from build123d import *

# Parameters (mm, degrees)
EXTRUDE_446_DEPTH      = 4.5
EXTRUDE_871_DEPTH      = 2.4
SKETCH_7_R             = 1.25
SKETCH_7_R_2           = 2.5
CUT_EXTRUDE_1133_DEPTH = 3
CHAMFER_1178_SIZE      = 1.5
EXTRUDE_START          = 4.5
SKETCH_8_R             = 2.85
SKETCH_8_R_2           = 1.25
EXTRUDE_1547_DEPTH     = 4.5
SKETCH_9_R             = 1.65
CUT_EXTRUDE_1826_DEPTH = 3
SKETCH_13_R            = 1.2
CUT_EXTRUDE_2013_DEPTH = 5
CUT_EXTRUDE_START      = -7
SKETCH_14_R            = 1.2
CUT_EXTRUDE_2216_DEPTH = 7
FILLET_2261_R          = 2


with BuildPart() as part:
    # Эскиз1 → Extrude 446 (new body)
    with BuildSketch(Plane.XY):
        with BuildLine():
            ThreePointArc((-48.184740917, 154.510381185), (-49.352687792, 153.677592944), (-49.8, 152.314674038))
            Line((-49.8, 152.314674038), (-49.8, 88.338690467))
            ThreePointArc((-49.8, 88.338690467), (-48.67998968, 86.364450269), (-46.41076143, 86.312966069))
            ThreePointArc((-46.41076143, 86.312966069), (-8.509697807, 97.629257558), (30.777662843, 93.040971394))
            ThreePointArc((30.777662843, 93.040971394), (32.846964094, 93.360279245), (33.8, 95.224598888))
            Line((33.8, 95.224598888), (33.8, 156.408950918))
            ThreePointArc((33.8, 156.408950918), (33.279664307, 157.865932371), (31.954091345, 158.663679516))
            ThreePointArc((31.954091345, 158.663679516), (-8.376811335, 161.632472551), (-48.184740917, 154.510381185))
        make_face()
        with BuildLine():
            Line((-47.4, 152.241091851), (-47.4, 88.505842281))
            ThreePointArc((-47.4, 88.505842281), (-8.703725392, 100.021444112), (31.4, 95.362907453))
            Line((31.4, 95.362907453), (31.4, 156.32706115))
            ThreePointArc((31.4, 156.32706115), (-8.256741868, 159.235474256), (-47.4, 152.241091851))
        make_face(mode=Mode.SUBTRACT)
    extrude(amount=-EXTRUDE_446_DEPTH)

    # Эскиз2 → Extrude 871 (add)
    with BuildSketch(Plane.XY):
        with BuildLine():
            Line((-52.4, 152.314674038), (-52.4, 88.338690467))
            ThreePointArc((-52.4, 88.338690467), (-50.013891057, 84.132700481), (-45.179448263, 84.023016749))
            ThreePointArc((-45.179448263, 84.023016749), (-8.283928985, 95.039078329), (29.961107796, 90.572522923))
            ThreePointArc((29.961107796, 90.572522923), (34.369619156, 91.252787475), (36.4, 95.224598888))
            Line((36.4, 95.224598888), (36.4, 156.408950918))
            ThreePointArc((36.4, 156.408950918), (35.291458741, 159.512954882), (32.467411995, 161.212503148))
            ThreePointArc((32.467411995, 161.212503148), (-8.511379087, 164.228987816), (-48.958795866, 156.992484917))
            ThreePointArc((-48.958795866, 156.992484917), (-51.447030513, 155.218283882), (-52.4, 152.314674038))
        make_face()
    extrude(amount=EXTRUDE_871_DEPTH)

    # Эскиз7 → Cut-Extrude 1133 (cut)
    with BuildSketch(Plane(origin=(0, 0, 0), x_dir=(-1, 0, 0), z_dir=(0, 0, -1))):
        with Locations((-29.451383649, 150.200294851)):
            Circle(SKETCH_7_R)
        with Locations((45.554851126, 150.200369953)):
            Circle(SKETCH_7_R)
        with Locations((45.55089452, 119.209232592)):
            Circle(SKETCH_7_R)
        with Locations((-29.454420734, 119.20872198)):
            Circle(SKETCH_7_R)
        with Locations((0, 155)):
            Circle(SKETCH_7_R_2)
    extrude(amount=-CUT_EXTRUDE_1133_DEPTH, mode=Mode.SUBTRACT)

    # Chamfer 1178
    chamfer_1178_edges = [part.edges().sort_by_distance(p)[0] for p in [
        (30.704420734, 119.20872198, 2.4),
        (-44.30089452, 119.209232592, 2.4),
        (-44.304851126, 150.200369953, 2.4),
        (30.701383649, 150.200294851, 2.4),
    ]]
    chamfer(chamfer_1178_edges, length=CHAMFER_1178_SIZE)

    # Эскиз8 → Extrude 1547 (add)
    # profile 1 of 4: a face of its own
    with BuildSketch(Plane(origin=(0, 0, 0), x_dir=(-1, 0, 0), z_dir=(0, 0, -1)).offset(EXTRUDE_START)):
        with Locations((-29.454420734, 119.20872198)):
            Circle(SKETCH_8_R)
        with Locations((-29.454420734, 119.20872198)):
            Circle(SKETCH_8_R_2, mode=Mode.SUBTRACT)
    # profile 2 of 4: a face of its own
    with BuildSketch(Plane(origin=(0, 0, 0), x_dir=(-1, 0, 0), z_dir=(0, 0, -1)).offset(EXTRUDE_START)):
        with Locations((-29.451383649, 150.200294851)):
            Circle(SKETCH_8_R)
        with Locations((-29.451383649, 150.200294851)):
            Circle(SKETCH_8_R_2, mode=Mode.SUBTRACT)
    # profile 3 of 4: a face of its own
    with BuildSketch(Plane(origin=(0, 0, 0), x_dir=(-1, 0, 0), z_dir=(0, 0, -1)).offset(EXTRUDE_START)):
        with Locations((45.55089452, 119.209232592)):
            Circle(SKETCH_8_R)
        with Locations((45.55089452, 119.209232592)):
            Circle(SKETCH_8_R_2, mode=Mode.SUBTRACT)
    # profile 4 of 4: a face of its own
    with BuildSketch(Plane(origin=(0, 0, 0), x_dir=(-1, 0, 0), z_dir=(0, 0, -1)).offset(EXTRUDE_START)):
        with Locations((45.554851126, 150.200369953)):
            Circle(SKETCH_8_R)
        with Locations((45.554851126, 150.200369953)):
            Circle(SKETCH_8_R_2, mode=Mode.SUBTRACT)
    extrude(amount=-EXTRUDE_1547_DEPTH)

    # Эскиз9 → Cut-Extrude 1826 (cut)
    with BuildSketch(Plane(origin=(0, 0, 0), x_dir=(-1, 0, 0), z_dir=(0, 0, -1))):
        with Locations((-28.380750513, 99.381741539)):
            Circle(SKETCH_9_R)
        with Locations((44.512478568, 93.278276156)):
            Circle(SKETCH_9_R)
        with Locations((-19.894937989, 155.969982116)):
            Circle(SKETCH_9_R)
        with Locations((18.78344627, 156.107738518)):
            Circle(SKETCH_9_R)
    extrude(amount=-CUT_EXTRUDE_1826_DEPTH, mode=Mode.SUBTRACT)

    # Эскиз13 → Cut-Extrude 2013 (cut)
    with BuildSketch(Plane.ZY.offset(49.8)):
        with Locations((-2.25, 144.314674038)):
            Circle(SKETCH_13_R)
        with Locations((-2.25, 91.438690467)):
            Circle(SKETCH_13_R)
    extrude(amount=-CUT_EXTRUDE_2013_DEPTH, mode=Mode.SUBTRACT)

    # Эскиз14 → Cut-Extrude 2216 (cut)
    with BuildSketch(Plane(origin=(33.8, 0, 0), x_dir=(0, 0, -1), z_dir=(1, 0, 0)).offset(CUT_EXTRUDE_START)):
        with Locations(Location((2.25, 144.314674038, 0), (0, 0, 180))):
            Circle(SKETCH_14_R)
        with Locations(Location((2.25, 103.724598888, 0), (0, 0, 90))):
            Circle(SKETCH_14_R)
    extrude(amount=CUT_EXTRUDE_2216_DEPTH, mode=Mode.SUBTRACT)

    # Fillet 2261
    # the kernel refuses this fillet: 2 mm, written as the material it adds along each edge
    with BuildSketch(Plane(origin=(-44.944004027, 152.98413823, -4.5), x_dir=(0.9624896485032316, 0.2713184043225332, 0), z_dir=(0, 0, 1))) as fillet_2261_piece_1:
        with BuildLine():
            CenterArc((3.479493085, -1.99987944), FILLET_2261_R, 89.370889764, 96.709553608)
            ThreePointArc((1.490744771, -2.21172878), (1.020072901, -0.920711328), (0, 0))
            ThreePointArc((0, 0), (1.750726367, 0.009611624), (3.501452734, 0))
        make_face()
    extrude(amount=4.5)
    with BuildSketch(Plane(origin=(31.4, 156.32706115, 0), x_dir=(0, -1, 0), z_dir=(0, 0, -1))) as fillet_2261_piece_2:
        with BuildLine():
            CenterArc((1.646899326, 2), FILLET_2261_R, 190.761817139, 79.238182861)
            ThreePointArc((-0.317924487, 1.626546679), (-0.16107556, 0.812860271), (0, 0))
            Line((0, 0), (1.646899326, 0))
        make_face()
    extrude(amount=4.5)
    with BuildSketch(Plane(origin=(31.4, 95.362907453, 0), x_dir=(0, 1, 0), z_dir=(0, 0, -1))) as fillet_2261_piece_3:
        with BuildLine():
            CenterArc((2.725225415, -2), FILLET_2261_R, 90, 106.685074195)
            ThreePointArc((0.809430773, -2.574221986), (0.413364342, -1.284391441), (0, 0))
            Line((0, 0), (2.725225415, 0))
        make_face()
    extrude(amount=4.5)
    with BuildSketch(Plane(origin=(-47.4, 88.505842281, 0), x_dir=(0.889056274455369, 0.45779792578335204, 0), z_dir=(0, 0, -1))) as fillet_2261_piece_4_section:
        with BuildLine():
            CenterArc((3.279293139, -1.999738508), FILLET_2261_R, 90.92652325, 116.318579463)
            Line((1.50118059, -2.91533436), (0, 0))
            ThreePointArc((0, 0), (1.623476393, -0.013126808), (3.246952786, 0))
        make_face()
    fillet_2261_piece_4 = extrude(amount=4.5, mode=Mode.PRIVATE)
    fillet_2261_piece_4 = fillet_2261_piece_4 - Plane(origin=(-46.674755075, 91.438690467, -2.25), x_dir=(0, 0, 1), z_dir=(-1, 0, 0)) * Cylinder(1.2, 22, mode=Mode.PRIVATE)
    add(fillet_2261_piece_4)


solid = part.part
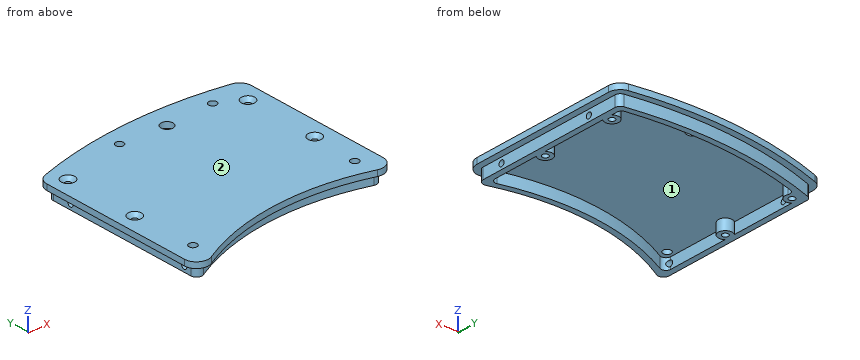
Verification items for the finished model (mm, model axes). Face numbers are marked on the shaded views. A direction names the side the tool comes from. Give positions to 0.01 mm unless a question says otherwise; leave off trailing zeros. Write each loop counter-clockwise with the first axis right and the second up, starting at its lowest first coordinate (ties: lowest second). Pieces come first, ordered by that corner, then holes. Notation, with made-up numbers: (85.5, -14) - (132.5, -14) arc R11 ccw to (132.5, 2) - close; hole circle Ø8 at (19, 35). An arc over 180 degrees is marked (long way). Answer as CSV lines item,"result". Start each with the question number.
1. Set-up check for the marked faces 1 and 2: record each of +Z, -Z, +X, -X, +Y, -Y from which the full face is reachable in a straight line by a thin tool's end or side.
2. Sectioned sample at A-A (x = 0). Record the boundary of the cut face in (y, z), then the cut area to 3 significant figures.
3. Sectioned sample at C-C (z = -2.25). Count the separate pieces of the cut face and the enclosed holes in it, then the cut area to 3 significant figures.
4. Depth check by flat-ended pin: pin 1 (2 mm diameter, centred on y = 144.31, z = -2.25, fed in from -X); pin 2 (1.3 mm diameter, centred on y = 136.5, z = -2.5, fed in from -X); pin 3 (2 mm diameter, centred on y = 136.5, z = -2, fed in from +X); pin 4 (4.5 mm diameter, centred on x = -18.78, y = 156.11, fed in from +Z). Enter the tip coordinate at first touch or a pass-through.
5. Thickness scan on line 1 (X direction, y = 140.5, z = -4); line 2 (X direction, y = 150.5, z = 1); line 3 (Y direction, x = 0, z = 0.8). Record the ranges inside material, lowest first.
6. Sectioned sample at B-B (y = 124.5). Record the boundary of the cut face in (x, z), then the cut area to 3 significant figures.
7. Sectioned sample at D-D (x = -33). Record the boundary of the cut face in (y, z), then the cut area to 3 significant figures.
Derived:
1,face 1,"-Z"
1,face 2,"+Z, +X, -X, +Y, -Y"
2,outline,"(95.4, 0) - (98, 0) - (98, -4.5) - (100.4, -4.5) - (100.4, 0) - (152.5, 0) - (152.5, 2.4) - (95.4, 2.4) - close; (157.5, 0) - (159.45, 0) - (159.45, -4.5) - (161.85, -4.5) - (161.85, 0) - (164.45, 0) - (164.45, 2.4) - (157.5, 2.4) - close"
2,area,"175 mm²"
3,separate pieces,"4"
3,enclosed holes,"4"
3,area,"758 mm²"
4,pin 1,"through"
4,pin 2,"x = -49.8"
4,pin 3,"x = 33.8"
4,pin 4,"z = 2.4"
5,line 1,"-49.8 to -47.4, 31.4 to 33.8"
5,line 2,"-52.4 to -46.87, -44.24 to 28.14, 30.77 to 36.4"
5,line 3,"95.4 to 152.5, 157.5 to 164.45"
6,outline,"(-52.4, 0) - (-49.8, 0) - (-49.8, -4.5) - (-47.4, -4.5) - (-47.4, 0) - (31.4, 0) - (31.4, -4.5) - (33.8, -4.5) - (33.8, 0) - (36.4, 0) - (36.4, 2.4) - (-52.4, 2.4) - close"
6,area,"235 mm²"
7,outline,"(89.51, 0) - (92.28, 0) - (92.28, -4.5) - (94.82, -4.5) - (94.82, 0) - (156, 0) - (156, -4.5) - (158.45, -4.5) - (158.45, 0) - (161.1, 0) - (161.1, 2.4) - (89.51, 2.4) - close"
7,area,"194 mm²"
